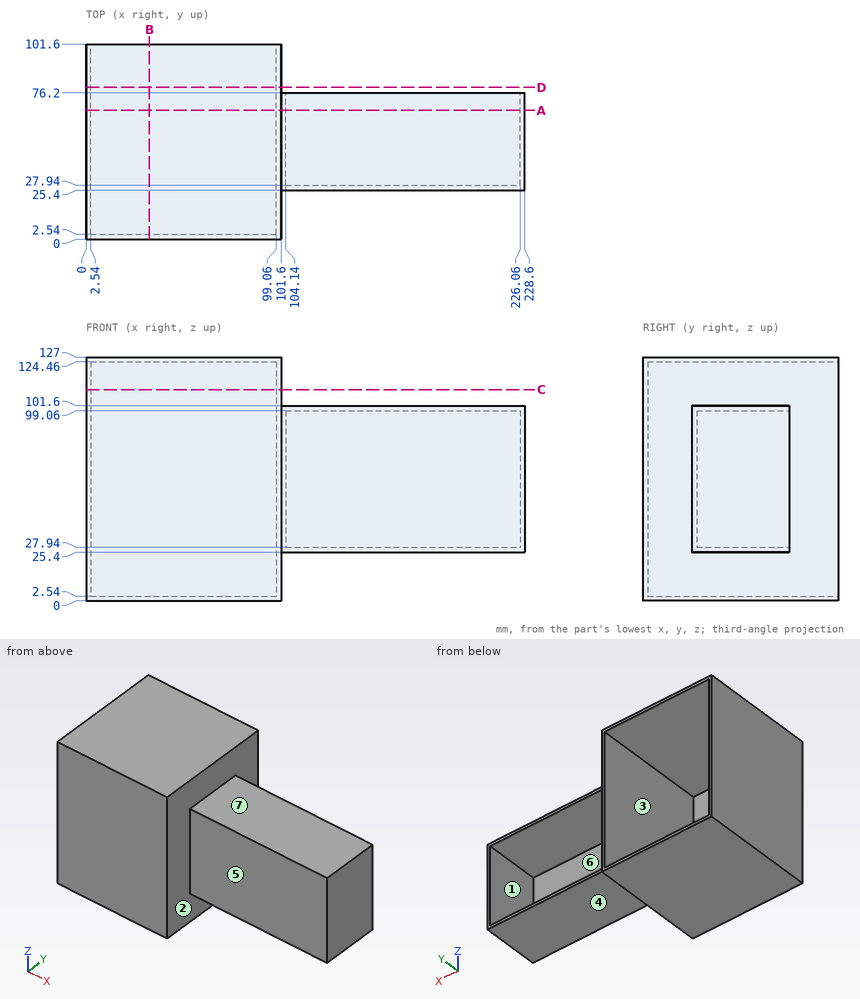
Verification items for this drawing (mm, ordinates from the low corner). A direction names the side the tool comes from. Round coordinates to 2 decimals unless told otherwise and drop trailing zeros. Loops run counter-clockwise (first coordinate to the right, second up) from the corner with the lowest first, then second, coordinate; pieces in that order, holes last. Notation, with made-up numbers: (68.5, 32) - (111.5, 32) arc R11 ccw to (111.5, 36) - close; hole circle Ø7 at (5, 15.5). An arc over 180 degrees is marked (long way). Answer as CSV lines item,"result". Start each with the question number.
Item 1: Release check for a two-part mould opening along Z. For the marked faces 1, 2, 3 and 4 record: +Z half, -Z half, draft (parallel to the pull), parting line (faces both ways), or undercut.
Item 2: Section check C-C (z = 110). Record the boundary of the cut face in (x, y).
Item 3: Section check B-B (x = 33). Record the boundary of the cut face in (y, z).
Item 4: Set-up check for the marked faces 5, 6 and 7: record each of +Z, -Z, +X, -X, +Y, -Y from which the full face is reachable in a straight line by a thin tool's end or side.
Item 5: Section check D-D (y = 79). Record the boundary of the cut face in (x, z), and give its area (3 significant figures).
Item 6: Scan lines: line 1 (Z direction, x = 43.5, y = 33); line 2 (X direction, y = 90.5, z = 44); line 3 (Z direction, x = 197, y = 31). Record each from-to range of solid material in increasing order. Write a range as [from, to].
Item 7: Section check A-A (y = 67). Record the boundary of the cut face in (x, z), and give its area (3 significant figures).
Item 8: Depth check by flat-ended pin: P1, Ø12, axis at x = 185, z = 96.5, coming from the +Y side; P2, Ø23, axis at x = 154.5, z = 48.5, coming from the -Y side; P3, Ø1.5, axis at y = 52.5, z = 105, coming from the +X side. Enter the tip coordinate at first touch or a pass-through.
Report:
1,face 1,"undercut"
1,face 2,"draft"
1,face 3,"undercut"
1,face 4,"-Z half"
2,outline,"(0, 0) - (101.6, 0) - (101.6, 101.6) - (99.06, 101.6) - (99.06, 2.54) - (2.54, 2.54) - (2.54, 101.6) - (0, 101.6) - close"
3,outline,"(0, 0) - (101.6, 0) - (101.6, 2.54) - (2.54, 2.54) - (2.54, 124.46) - (101.6, 124.46) - (101.6, 127) - (0, 127) - close"
4,face 5,"+Z, -Z, +X, -Y"
4,face 6,"+Y"
4,face 7,"+Z, +X, +Y, -Y"
5,outline,"(0, 0) - (101.6, 0) - (101.6, 127) - (0, 127) - close; hole (2.54, 2.54) - (99.06, 2.54) - (99.06, 124.46) - (2.54, 124.46) - close"
5,area,"1,140 mm2"
6,line 1,"z = [0, 2.54], [124.46, 127]"
6,line 2,"x = [0, 2.54], [99.06, 101.6]"
6,line 3,"z = [25.4, 27.94], [99.06, 101.6]"
7,outline,"(0, 0) - (101.6, 0) - (101.6, 25.4) - (228.6, 25.4) - (228.6, 101.6) - (101.6, 101.6) - (101.6, 127) - (0, 127) - close; hole (2.54, 2.54) - (99.06, 2.54) - (99.06, 124.46) - (2.54, 124.46) - close; hole (104.14, 27.94) - (226.06, 27.94) - (226.06, 99.06) - (104.14, 99.06) - close"
7,area,"2,140 mm2"
8,P1,"stops at y = 76.2"
8,P2,"stops at y = 25.4"
8,P3,"stops at x = 101.6"
